Input: part model. Units: mm. Frame: model coordinates. A direction names the side the tool comes from. Give positions to 0.01 mm unless a question says otherwise; leave off trailing zeros. Loops run counter-clockwise (first coordinate to the right, second up) from the corner with the lowest first, then second, coordinate; pieces in that order, holes last. Notation, with made-up numbers: M -14,-1 L -4,-1 A27 cw -4,36 Z; hole C 81,47 d9. An arc over 180 degrees is marked long. Use CSV: the item, a comma, the result in double quotes. Start each with the question number.
from build123d import *

# Parameters (mm, degrees)
SKETCH1_W           = 111.1
SKETCH1_H           = 51.3
BOSS_EXTRUDE1_DEPTH = 5
SKETCH9_W           = 5
SKETCH9_H           = 4
BOSS_EXTRUDE5_DEPTH = 3
SKETCH10_R          = 2.55
SKETCH10_W          = 10
SKETCH10_H          = 4.5
CUT_EXTRUDE1_DEPTH  = 10
SKETCH11_R          = 1.8
CUT_EXTRUDE2_DEPTH  = 3
FILLET1_R           = 2


with BuildPart() as part:
    # Sketch1 → Boss-Extrude1 (new body)
    with BuildSketch(Plane(origin=(0, 0, 0), x_dir=(1, 0, 0), z_dir=(0, 1, 0))):
        Rectangle(SKETCH1_W, SKETCH1_H)
    extrude(amount=BOSS_EXTRUDE1_DEPTH)

    # Sketch9 → Boss-Extrude5 (add)
    with BuildSketch(Plane.XZ):
        with Locations((-48.05, -20.65)):
            Rectangle(SKETCH9_W, SKETCH9_H)
        with Locations((48.05, -20.65)):
            Rectangle(SKETCH9_W, SKETCH9_H)
    extrude(amount=BOSS_EXTRUDE5_DEPTH)

    # Sketch10 → Cut-Extrude1 (cut)
    with BuildSketch(Plane(origin=(0, 5, 0), x_dir=(1, 0, 0), z_dir=(0, 1, 0))):
        with Locations(Location((-36.275, 17.65, 0), (0, 0, 270))):
            Circle(SKETCH10_R)
        with Locations(Location((16.275, 17.65, 0), (0, 0, 270))):
            Circle(SKETCH10_R)
        with Locations((-20.275, 17.65)):
            Rectangle(SKETCH10_W, SKETCH10_H)
        with Locations((32.275, 17.65)):
            Rectangle(SKETCH10_W, SKETCH10_H)
    extrude(amount=-CUT_EXTRUDE1_DEPTH, mode=Mode.SUBTRACT)

    # Sketch11 → Cut-Extrude2 (cut)
    with BuildSketch(Plane.XZ):
        with Locations(Location((-30.025, -17.65, 0), (0, 0, 270))):
            Circle(SKETCH11_R)
        with Locations(Location((-10.525, -17.65, 0), (0, 0, 270))):
            Circle(SKETCH11_R)
        with Locations(Location((22.525, -17.65, 0), (0, 0, 270))):
            Circle(SKETCH11_R)
        with Locations(Location((42.025, -17.65, 0), (0, 0, 270))):
            Circle(SKETCH11_R)
    extrude(amount=-CUT_EXTRUDE2_DEPTH, mode=Mode.SUBTRACT)

    # Fillet1
    fillet1_edges = [part.edges().sort_by_distance(p)[0] for p in [
        (-55.55, 2.5, -25.65),
        (55.55, 2.5, -25.65),
        (55.55, 2.5, 25.65),
        (-55.55, 2.5, 25.65),
    ]]
    fillet(fillet1_edges, radius=FILLET1_R)


solid = part.part
Item 1: Set-up query: faces 1 (the cylindrical face through (-11.62, 1.48, -16.22)), 2 (the flat face through (27.275, 3, -18)), 3 (the cylindrical face through (-54.98, 2.54, 25.05)), 4 (the flat face through (-45.55, -1, -21)), 5 (the flat face through (-1, 5, 0)). Return all of +Z, -Z, +X, -X, +Y, -Y with unobstructed straight access to the full face (end or side cutting, diameter ignored); none if empty.
Item 2: Section C-C (z = -17.65). State how many separate pieces and enclosed holes the cut face has, then the cut area to 3 significant figures.
Item 3: Section D-D (x = 6). Output: boundary loops of the cut face in (y, z), then the cut area to 4 significant figures.
Item 4: Section B-B (y = -1). Output: boundary loops of the cut face in (x, z).
Item 5: Mould query, pull axis X, two halves, no side actions, for faces 6 (the flat face through (-1, 2, 25.65)), 7 (the flat face through (55.55, 2, 0)), 8 (the cylindrical face through (-37.83, 2.54, -19.67)). Classes: +X half, -X half, draft (parallel to the pull), parting line (faces both ways), or undercut.
Item 6: Section A-A (x = -18). Output: boundary loops of the cut face in (y, z).
Item 7: Material intervals for line 1 (X direction, y = 3.6, z = -17.65) (3 decimals); line 2 (Y direction, x = 4, z = -19); line 3 (Z direction, x = 34, y = 2), sorted ascending.
Item 8: First-contact query: pin 1 Ø1.1 at (x, z) = (21.5, -18) entering from -Y; pin 2 Ø4 at (y, z) = (-1.5, -0.5) entering from -X; pin 3 Ø6 at (x, z) = (-22, -17) entering from -Y; pin 4 Ø1.5 at (x, y) = (48.5, -1.5) entering from -Z. Flat tips, straight axial feed; report the tip coordinate or a pass-through.
Recorded:
1,face 1,"-Y"
1,face 2,"+Y, -Y"
1,face 3,"+Z, -X, +Y, -Y"
1,face 4,"+Z, -Z, -Y"
1,face 5,"+Z, -Z, +X, -X, +Y"
2,separate pieces,"5"
2,enclosed holes,"0"
2,area,"361 mm²"
3,outline,"M 0,-25.65 L 5,-25.65 L 5,25.65 L 0,25.65 Z"
3,area,"256.5 mm²"
4,outline,"M -50.55,-22.65 L -45.55,-22.65 L -45.55,-18.65 L -50.55,-18.65 Z; M 45.55,-22.65 L 50.55,-22.65 L 50.55,-18.65 L 45.55,-18.65 Z"
5,face 6,"draft"
5,face 7,"+X half"
5,face 8,"undercut"
6,outline,"M 0,-25.65 L 5,-25.65 L 5,-19.9 L 0,-19.9 Z; M 0,-15.4 L 5,-15.4 L 5,25.65 L 0,25.65 Z"
7,line 1,"-55.55 to -38.825, -33.725 to -25.275, -15.275 to 13.725, 18.825 to 27.275, 37.275 to 55.55"
7,line 2,"0 to 5"
7,line 3,"-25.65 to -19.9, -15.4 to 25.65"
8,pin 1,"y = 3"
8,pin 2,"x = -55.55"
8,pin 3,"y = 0"
8,pin 4,"z = -22.65"
